Autodesk Inventor part; units mm, degrees
ref_plane "YZ Plane" through (0, 0, 0) normal (1, 0, 0) x (0, 1, 0)
ref_plane "XZ Plane" through (0, 0, 0) normal (0, 1, 0) x (-1, 0, 0)
ref_plane "XY Plane" through (0, 0, 0) normal (0, 0, 1) x (1, 0, 0)
sketch "Sketch1" plane through (0, 0, 0) normal (0, 0, 1) x (1, 0, 0)
  line L0 (-17.75, -20.25) -> (17.75, -20.25)
  line L1 (17.75, -20.25) -> (17.75, 20.25)
  line L2 (17.75, 20.25) -> (-17.75, 20.25)
  line L3 (-17.75, 20.25) -> (-17.75, -20.25)
  line L4 (-17.75, -20.25) -> (17.75, 20.25) construction
  line L5 (17.75, -20.25) -> (-17.75, 20.25) construction
  point P0 (0, 0)
  dimension "d0" = 35.5
  dimension "d1" = 40.5
extrude "Plate1" add sketch "Sketch1" along normal blind 1.5
sketch "Sketch2" plane through (-17.75, 18.75, 0) normal (0, 1, 0) x (-1, 0, 0)
  line L0 (-35.5, 0) -> (0, 0)
  line L1 (0, 0) -> (0, 10)
  line L2 (0, 10) -> (-35.5, 10)
  line L3 (-35.5, 10) -> (-35.5, 0)
edge flange "Flange1" height 10 angle 90 thickness 1.5 bend radius 0.31 thickness toward (0, 1, 0) relief tear relief width 1.5 relief depth 0.75 corner gap 0.31 corner form 0 edges at (0, 20.25, 1.5) (0, -20.25, 1.5) wall of the first edge with corners at (17.75, 18.75, 0) (-17.75, 18.75, 0) (-17.75, 18.75, 10) (17.75, 18.75, 10)
bend "Bend1"
corner "Corner1"
sketch "Sketch3" plane through (-17.75, 20.25, 10) normal (0, 1, 0) x (1, 0, 0)
  line L0 (35.5, 8.19) -> (0, 8.19)
  line L1 (0, 0) -> (0, 8.19)
  line L2 (35.5, 0) -> (0, 0)
  line L3 (35.5, 8.19) -> (35.5, 0)
  point P0 (17.75, 10)
  point P1 (8, 4.095)
  point P2 (27.5, 4.095)
  point P3 (0, 4.095)
  point P4 (35.5, 4.095)
  dimension "d13" = 8
  dimension "d14" = 8
hole "Hole1" at (-9.75, 20.25, 5.905) at (9.75, 20.25, 5.905) direction (0, -1, 0) diameter 1.567 depth 1.5
sketch "Sketch4" plane through (-17.75, -20.25, 10) normal (0, -1, 0) x (1, 0, 0)
  circle A0 centre (27.5, -4.095) radius 0.7835
  circle A1 centre (8, -4.095) radius 0.7835
  point P0 (17.75, -10)
hole "Hole2" at (9.75, -20.25, 5.905) at (-9.75, -20.25, 5.905) direction (0, 1, 0) diameter 1.567 depth 1.5
fillet "Corner Round1" radius 2 4 edges at (17.75, 19.5, 10) (-17.75, 19.5, 10) (17.75, -19.5, 10) (-17.75, -19.5, 10)
equation "\"d20\" = Thickness"
equation "\"d2\" = Thickness"
equation "\"d3\" = BendReliefWidth"
equation "\"d4\" = BendReliefDepth"
equation "\"d5\" = MinimumRemnant"
equation "\"d6\" = TransitionRadius"
equation "\"d9\" = BendRadius"
equation "\"d10\" = CornerReliefSize"
equation "\"d11\" = GapSize"
equation "\"d12\" = JacobiRadiusSize"
equation "\"BendReliefWidth\" = Thickness"
equation "\"BendReliefDepth\" = 0.5 * Thickness"
equation "\"CornerReliefSize\" = 4 * Thickness"
equation "\"MinimumRemnant\" = 2 * Thickness"
equation "\"TransitionRadius\" = BendRadius"
equation "\"JacobiRadiusSize\" = BendRadius"
equation "\"GapSize\" = Thickness"
properties part number "ㄷ_frame_3" material "Aluminum 6061"
Geometry check sheet. Reference: the model listing, model coordinates, mm. A direction names the side the tool comes from. Give positions to 0.01 mm unless a question says otherwise; leave off trailing zeros. Write each loop counter-clockwise with the first axis right and the second up, starting at its lowest first coordinate (ties: lowest second). Pieces come first, ordered by that corner, then holes. Notation, with made-up numbers: M -16.75,55 L 15.25,55 A30 ccw 15.25,92 Z; hole C -33.75,86 d2. An arc over 180 degrees is marked long. One line per question, with ' | ' between items.
1. Cross-section at C-C (x = -3). Enter the section's corners in (y, z), plus the area to 3 significant figures.
Ans:
outline: M -20.25,1.81 A1.81 ccw -18.44,0 L 18.44,0 A1.81 ccw 20.25,1.81 L 20.25,10 L 18.75,10 L 18.75,1.81 A0.31 cw 18.44,1.5 L -18.44,1.5 A0.31 cw -18.75,1.81 L -18.75,10 L -20.25,10 Z | area: 84.9 mm2
2. Set-up check for faces 1 (the face through (17.18, -19.51, 9.4)), 2 (the face through (0, 18.75, 6)): record each of +Z, -Z, +X, -X, +Y, -Y from which the full face is reachable in a straight line by a thin tool's end or side.
Ans:
face 1: +Z, +X, +Y, -Y | face 2: +Z, +X, -X
3. Cross-section at D-D (z = 5.75). Enter the section's corners in (x, y), plus the area to 3 significant figures.
Ans:
outline: M -17.75,-20.25 L -10.52,-20.25 L -10.52,-18.75 L -17.75,-18.75 Z; M -17.75,18.75 L -10.52,18.75 L -10.52,20.25 L -17.75,20.25 Z; M -8.98,-20.25 L 8.98,-20.25 L 8.98,-18.75 L -8.98,-18.75 Z; M -8.98,18.75 L 8.98,18.75 L 8.98,20.25 L -8.98,20.25 Z; M 10.52,-20.25 L 17.75,-20.25 L 17.75,-18.75 L 10.52,-18.75 Z; M 10.52,18.75 L 17.75,18.75 L 17.75,20.25 L 10.52,20.25 Z | area: 97.3 mm2
4. Cross-section at A-A (x = 9.75). Enter the section's corners in (y, z), plus the area to 3 significant figures.
Ans:
outline: M -20.25,1.81 A1.81 ccw -18.44,0 L 18.44,0 A1.81 ccw 20.25,1.81 L 20.25,5.12 L 18.75,5.12 L 18.75,1.81 A0.31 cw 18.44,1.5 L -18.44,1.5 A0.31 cw -18.75,1.81 L -18.75,5.12 L -20.25,5.12 Z; M -20.25,6.69 L -18.75,6.69 L -18.75,10 L -20.25,10 Z; M 18.75,6.69 L 20.25,6.69 L 20.25,10 L 18.75,10 Z | area: 80.2 mm2
5. Mould release check, pull along Z, two halves, no side actions. Record for faces 3 (the face through (10.445, -19.49, 5.543)), 4 (the face through (0, -20.25, 6)), 5 (the face through (-0.25, 19.73, 0.54)): released by +Z, released by -Z, zero draft, split by the parting line, or undercut.
Ans:
face 3: undercut | face 4: zero draft | face 5: released by -Z
6. Cross-section at B-B (z = 3.75). Enter the section's corners in (x, y).
Ans:
outline: M -17.75,-20.25 L 17.75,-20.25 L 17.75,-18.75 L -17.75,-18.75 Z; M -17.75,18.75 L 17.75,18.75 L 17.75,20.25 L -17.75,20.25 Z
7. Gauge pin test, flat end, axial feed: pin 1 (1.5 mm diameter, centred on y = -1.5, z = 3.5, fed in from -X). Record the tip position at first contact, or that the pin passes through.
Ans:
pin 1: through
8. Scan lines: line 1 along Y through (x, z) = (5, 4.25); line 2 along Z through (x, y) = (-15, 8); line 3 along Z through (x, y) = (9.75, 19.25). Record each from-to range of solid material in increasing order. Write a range as from..to.
Ans:
line 1: -20.25..-18.75, 18.75..20.25 | line 2: 0..1.5 | line 3: 0.19..5.12, 6.69..10
